Geometry: final body of the model. Coordinates: model frame, mm. Round coordinates to 2 decimals unless told otherwise and drop trailing zeros. Loops run counter-clockwise (first coordinate to the right, second up) from the corner with the lowest first, then second, coordinate; pieces in that order, holes last. Notation, with made-up numbers: (79.25, 2.25) - (85.25, 2.25) arc R29 cw to (85.25, 27.25) - close; hole circle Ø11 at (86, -12.5). An arc over 180 degrees is marked (long way). Write item = value, one per line. Start each with the question number.
Item 1: Section C-C (y = 1.05). Return loops of the section in (x, z), plus the area to 3 significant figures.
Item 2: Section D-D (z = 6.5). Return loops of the section in (x, y).
Item 3: Line query: line 1 (Z direction, x = -6.5, y = 0.55); line 2 (Z direction, x = -7.5, y = 1); line 3 (X direction, y = 1, z = 7). Output: solid intervals per line, ascending. Write a range as from..to.
Item 4: Section B-B (z = -7). Return loops of the section in (x, y).
Item 5: Draft query along X for faces 1 (the cylindrical face through (-8.73, 0.63, 9.43)), 2 (the flat face through (0, 1, 14)), 3 (the flat face through (-13.5, 1, 0)). Return one class per face: pulls with the +X half, pulls with the -X half, needs draft (parallel to the pull), parting line crosses it, or undercut.
Item 6: Section A-A (x = -6.5). Return loops of the section in (y, z), plus the area to 3 significant figures.
Autodesk Inventor part; units mm, degrees
ref_plane "YZ Plane" through (0, 0, 0) normal (1, 0, 0) x (0, 1, 0)
ref_plane "XZ Plane" through (0, 0, 0) normal (0, 1, 0) x (-1, 0, 0)
ref_plane "XY Plane" through (0, 0, 0) normal (0, 0, 1) x (1, 0, 0)
sketch "Sketch1" plane through (0, 0, 0) normal (0, 1, 0) x (-1, 0, 0)
  line L0 (-13.5, 14) -> (13.5, 14)
  line L1 (13.5, 14) -> (13.5, -14)
  line L2 (13.5, -14) -> (-13.5, -14)
  line L3 (-13.5, -14) -> (-13.5, 14)
  line L4 (-13.5, 14) -> (13.5, -14) construction
  line L5 (13.5, 14) -> (-13.5, -14) construction
  point P0 (0, 0)
  dimension "d0" = 27
  dimension "d1" = 28
extrude "Extrusion1" add sketch "Sketch1" along normal blind 1.25
sketch "Sketch2" plane through (0, 0, 0) normal (0, -1, 0) x (1, 0, 0)
  circle A0 centre (-6.5, 7) radius 3.3
  circle A1 centre (-6.5, -7) radius 3.3
  line L0 (-13.5, 14) -> (-13.5, -14)
  line L1 (19.5, -14) -> (-13.5, -14)
  line L2 (19.5, 14) -> (19.5, -14)
  line L3 (-13.5, 14) -> (19.5, 14)
  point P0 (0, 0)
hole "Hole1" at (-6.5, 0, 7) at (-6.5, 0, -7) direction (0, 1, 0) diameter 6.6 depth 8 tip angle 118
properties part number "SP37V1 Suplemento Refuerzo"
Taken from the geometry:
q1.outline = (-13.5, -14) - (13.5, -14) - (13.5, 14) - (-13.5, 14) - close; hole circle Ø6.6 at (-6.5, -7); hole circle Ø6.6 at (-6.5, 7)
q1.area = 688 mm^2
q2.outline = (-13.5, 0) - (-9.76, 0) - (-9.76, 1.25) - (-13.5, 1.25) - close; (-3.24, 0) - (13.5, 0) - (13.5, 1.25) - (-3.24, 1.25) - close
q3.line_1 = -14..-10.3, -3.7..3.7, 10.3..14
q3.line_2 = -14..-10.14, -3.86..3.86, 10.14..14
q3.line_3 = -13.5..-9.8, -3.2..13.5
q4.outline = (-13.5, 0) - (-9.8, 0) - (-9.8, 1.25) - (-13.5, 1.25) - close; (-3.2, 0) - (13.5, 0) - (13.5, 1.25) - (-3.2, 1.25) - close
q5.face_1 = undercut
q5.face_2 = needs draft
q5.face_3 = pulls with the -X half
q6.outline = (0, -14) - (1.25, -14) - (1.25, -10.3) - (0, -10.3) - close; (0, -3.7) - (1.25, -3.7) - (1.25, 3.7) - (0, 3.7) - close; (0, 10.3) - (1.25, 10.3) - (1.25, 14) - (0, 14) - close
q6.area = 18.5 mm^2
